Autodesk Fusion 360 part; units mm, degrees
sketch "Sketch1" plane through (0, 0, 0) normal (0, 0, 1) x (1, 0, 0)
  line L0 (68.541, -12.5) -> (-110, -12.5) construction
  line L1 (-20.75, -50) -> (-20.75, 25) construction
  point P0 (-20.75, -12.5)
sketch "Sketch2" plane through (0, 0, 0) normal (0, 0, 1) x (1, 0, 0)
  line L0 (54.25, 7.5) -> (-95.75, 7.5)
  line L1 (-95.75, 7.5) -> (-95.75, -32.5)
  line L2 (-95.75, -32.5) -> (54.25, -32.5)
  line L3 (54.25, -32.5) -> (54.25, 7.5)
  line L4 (54.25, 7.5) -> (-95.75, -32.5) construction
  line L5 (-95.75, 7.5) -> (54.25, -32.5) construction
  line L6 (26.6666, -12.5) -> (38.5, -12.5) construction
  circle A0 centre (32.5833, -12.5) radius 2.75
  line L7 (14, -12.5) -> (2.2, -12.5) construction
  circle A1 centre (8.1, -12.5) radius 2.75
  line L8 (-49.1, -12.5) -> (-52.4, -12.5) construction
  circle A2 centre (-52.4, -12.5) radius 2.75
  line L9 (-73.1, -12.5) -> (-69.8, -12.5) construction
  circle A3 centre (-69.8, -12.5) radius 2.75
  point P0 (-20.75, -12.5)
  dimension "d1" = 150
  dimension "d2" = 40
  dimension "d3" = 5.5
  dimension "d4" = 5.5
  dimension "d5" = 3.3
  dimension "d6" = 5.5
  dimension "d7" = 3.3
  dimension "d8" = 5.5
extrude "Extrude1" add sketch "Sketch2" along normal blind 2.5
sketch "Sketch3" plane through (0, 0, 2.5) normal (0, 0, 1) x (-1, 0, 0)
  circle A0 centre (-32.5833, 12.5) radius 2.75
  circle A1 centre (69.8, 12.5) radius 2.75
  circle A2 centre (-8.1, 12.5) radius 2.75
  circle A3 centre (52.4, 12.5) radius 2.75
  line L0 (-54.25, 32.5) -> (-54.25, -7.5)
  line L1 (-54.25, -7.5) -> (95.75, -7.5)
  line L2 (95.75, -7.5) -> (95.75, 32.5)
  line L3 (95.75, 32.5) -> (-54.25, 32.5)
sketch "Sketch4" plane through (0, 0, 2.5) normal (0, 0, 1) x (-1, 0, 0)
  line L0 (-29.8338, 12.5) -> (-35.3337, 12.5) construction
  line L1 (-39.2087, 4.875) -> (-25.9587, 4.875)
  line L2 (-25.9587, 4.875) -> (-25.9587, 20.125)
  line L3 (-25.9587, 20.125) -> (-39.2087, 20.125)
  line L4 (-39.2087, 20.125) -> (-39.2087, 4.875)
  line L5 (-39.2087, 4.875) -> (-25.9587, 20.125) construction
  line L6 (-25.9587, 4.875) -> (-39.2087, 20.125) construction
  line L7 (-41.2087, 2.875) -> (-23.9587, 2.875)
  line L8 (-23.9587, 2.875) -> (-23.9587, 22.125)
  line L9 (-23.9587, 22.125) -> (-41.2087, 22.125)
  line L10 (-41.2087, 22.125) -> (-41.2087, 2.875)
  line L11 (-41.2087, 2.875) -> (-23.9587, 22.125) construction
  line L12 (-23.9587, 2.875) -> (-41.2087, 22.125) construction
  line L13 (-39.2087, 12.5) -> (-39.2087, 9)
  line L14 (-39.2087, 9) -> (-41.2087, 9)
  line L15 (-41.2087, 9) -> (-41.2087, 16)
  line L16 (-41.2087, 16) -> (-39.2087, 16)
  line L17 (-39.2087, 16) -> (-39.2087, 12.5)
  line L18 (-5.35, 12.5) -> (-10.85, 12.5) construction
  line L19 (-14.725, 4.875) -> (-1.475, 4.875)
  line L20 (-1.475, 4.875) -> (-1.475, 20.125)
  line L21 (-1.475, 20.125) -> (-14.725, 20.125)
  line L22 (-14.725, 20.125) -> (-14.725, 4.875)
  line L23 (-14.725, 4.875) -> (-1.475, 20.125) construction
  line L24 (-1.475, 4.875) -> (-14.725, 20.125) construction
  line L25 (-16.725, 2.875) -> (0.525, 2.875)
  line L26 (0.525, 2.875) -> (0.525, 22.125)
  line L27 (0.525, 22.125) -> (-16.725, 22.125)
  line L28 (-16.725, 22.125) -> (-16.725, 2.875)
  line L29 (-16.725, 2.875) -> (0.525, 22.125) construction
  line L30 (0.525, 2.875) -> (-16.725, 22.125) construction
  line L31 (-1.475, 16) -> (-1.475, 9)
  line L32 (0.525, 16) -> (0.525, 9)
  line L33 (0.525, 9) -> (-1.475, 9)
  line L34 (0.525, 16) -> (-1.475, 16)
  line L35 (55.15, 12.5) -> (49.65, 12.5) construction
  line L36 (45.775, 4.875) -> (59.025, 4.875)
  line L37 (59.025, 4.875) -> (59.025, 20.125)
  line L38 (59.025, 20.125) -> (45.775, 20.125)
  line L39 (45.775, 20.125) -> (45.775, 4.875)
  line L40 (45.775, 4.875) -> (59.025, 20.125) construction
  line L41 (59.025, 4.875) -> (45.775, 20.125) construction
  line L42 (61.025, 22.125) -> (43.775, 22.125)
  line L43 (43.775, 22.125) -> (43.775, 2.875)
  line L44 (43.775, 2.875) -> (61.025, 2.875)
  line L45 (61.025, 22.125) -> (43.775, 2.875) construction
  line L46 (43.775, 22.125) -> (61.025, 2.875) construction
  line L47 (72.55, 12.5) -> (67.05, 12.5) construction
  line L48 (63.175, 4.875) -> (76.425, 4.875)
  line L49 (76.425, 4.875) -> (76.425, 20.125)
  line L50 (76.425, 20.125) -> (63.175, 20.125)
  line L51 (63.175, 20.125) -> (63.175, 4.875)
  line L52 (63.175, 4.875) -> (76.425, 20.125) construction
  line L53 (76.425, 4.875) -> (63.175, 20.125) construction
  line L54 (61.175, 2.875) -> (78.425, 2.875)
  line L55 (78.425, 2.875) -> (78.425, 22.125)
  line L56 (78.425, 22.125) -> (61.175, 22.125)
  line L57 (61.175, 2.875) -> (78.425, 22.125) construction
  line L58 (78.425, 2.875) -> (61.175, 22.125) construction
  line L59 (61.175, 2.875) -> (61.025, 2.875)
  line L60 (61.175, 22.125) -> (61.025, 22.125)
  line L61 (43.775, 16) -> (43.775, 9)
  line L62 (45.775, 16) -> (45.775, 9)
  line L63 (45.775, 9) -> (43.775, 9)
  line L64 (45.775, 16) -> (43.775, 16)
  line L65 (76.425, 16) -> (76.425, 9)
  line L66 (78.425, 16) -> (78.425, 9)
  line L67 (78.425, 9) -> (76.425, 9)
  line L68 (76.425, 16) -> (78.425, 16)
  point P0 (-32.5837, 12.5)
  point P1 (-32.5837, 12.5)
  point P2 (-8.1, 12.5)
  point P3 (-8.1, 12.5)
  point P4 (-1.475, 12.5)
  point P5 (0.525, 12.5)
  point P6 (52.4, 12.5)
  point P7 (52.4, 12.5)
  point P8 (69.8, 12.5)
  point P9 (69.8, 12.5)
  point P10 (43.775, 12.5)
  point P11 (45.775, 12.5)
  point P12 (76.425, 12.5)
  point P13 (78.425, 12.5)
  dimension "d11" = 13.25
  dimension "d12" = 15.25
  dimension "d13" = 17.25
  dimension "d14" = 19.25
  dimension "d15" = 3.5
  dimension "d16" = 7
  dimension "d17" = 13.25
  dimension "d18" = 15.25
  dimension "d19" = 17.25
  dimension "d20" = 19.25
  dimension "d21" = 7
  dimension "d22" = 7
  dimension "d23" = 13.25
  dimension "d24" = 15.25
  dimension "d25" = 17.25
  dimension "d26" = 19.25
  dimension "d27" = 13.25
  dimension "d28" = 15.25
  dimension "d29" = 17.25
  dimension "d30" = 19.25
  dimension "d31" = 7
  dimension "d32" = 7
  dimension "d33" = 7
  dimension "d34" = 7
extrude "Extrude2" add sketch "Sketch4" along normal blind 12 contours L1 L2 L3 L4 L7 L8 L9 L10 L14 L16 | L19 L20 L21 L22 L25 L26 L27 L28 L33 L34 | L36 L37 L38 L39 L42 L43 L44 L48 L49 L50 L51 L54 L55 L56 L59 L60 L63 L64 L67 L68
sketch "Sketch5" plane through (0, 0, 2.5) normal (0, 0, 1) x (-1, 0, 0)
sketch "Sketch7" plane through (54.25, 0, 0) normal (1, 0, 0) x (0, 1, 0)
  line L0 (-32.5, 0) -> (7.5, 0)
  line L1 (7.5, 0) -> (7.5, 2.5)
  line L2 (7.5, 2.5) -> (-32.5, 2.5)
  line L3 (-32.5, 2.5) -> (-32.5, 0)
  line L4 (-25, 2.5) -> (0, 2.5)
  line L5 (-21.5, 2.5) -> (-3.5, 2.5)
  line L6 (-12.5, 7.5) -> (-3.5, 7.5)
  line L7 (-3.5, 7.5) -> (0, 2.5)
  line L8 (-12.5, 7.5) -> (-21.5, 7.5)
  line L9 (-21.5, 7.5) -> (-25, 2.5)
  line L10 (-12.5, 2.5) -> (-12.5, 7.5) construction
  circle A0 centre (-12.5, 5) radius 1.25
  point P0 (-12.5, 2.5)
  point P1 (-12.5, 2.5)
  dimension "d39" = 25
  dimension "d40" = 18
  dimension "d41" = 2.5
extrude "Extrude3" add sketch "Sketch7" against normal blind 2.5 contours L2 L4 L5 L6 L7 L8 L9
sketch "Sketch8" plane through (-95.75, 0, 0) normal (-1, 0, 0) x (0, -1, 0)
  line L0 (-7.5, 0) -> (32.5, 0)
  line L1 (32.5, 0) -> (32.5, 2.5)
  line L2 (32.5, 2.5) -> (-7.5, 2.5)
  line L3 (-7.5, 2.5) -> (-7.5, 0)
  line L4 (0, 2.5) -> (25, 2.5)
  line L5 (3.5, 7.5) -> (21.5, 7.5)
  line L6 (3.5, 7.5) -> (0, 2.5)
  line L7 (21.5, 7.5) -> (25, 2.5)
  circle A0 centre (12.5, 5) radius 1.25
  point P0 (12.5, 2.5)
  dimension "d44" = 25
  dimension "d46" = 18
  dimension "d47" = 2.5
extrude "Extrude4" add sketch "Sketch8" against normal blind 2.5 contours L2 L4 L5 L6 L7
fillet "Fillet1" radius 1 4 edges at (-94.5, -21.5, 7.5) (-94.5, -25, 2.5) (-94.5, -3.5, 7.5) (-94.5, 0, 2.5)
fillet "Fillet2" radius 1 4 edges at (53, -25, 2.5) (53, -21.5, 7.5) (53, -3.5, 7.5) (53, 0, 2.5)
fillet "Fillet3" radius 0.5 5 edges at (41.2087, -19.0625, 2.5) (32.5837, -22.125, 2.5) (41.2087, -5.9375, 2.5) (32.5837, -2.875, 2.5) (23.9587, -12.5, 2.5)
fillet "Fillet4" radius 0.5 15 edges at (16.725, -12.5, 2.5) (8.1, -2.875, 2.5) (8.1, -22.125, 2.5) (-0.525, -5.9375, 2.5) (-0.525, -19.0625, 2.5) (-52.4, -22.125, 2.5) (-61.1, -22.125, 2.5) (-69.8, -22.125, 2.5) (-78.425, -19.0625, 2.5) (-78.425, -5.9375, 2.5) (-43.775, -19.0625, 2.5) (-43.775, -5.9375, 2.5) (-69.8, -2.875, 2.5) (-61.1, -2.875, 2.5) (-52.4, -2.875, 2.5)
fillet "Fillet5" radius 1 8 edges at (-45.775, -16, 8.5) (-45.775, -9, 8.5) (-76.425, -9, 8.5) (-76.425, -16, 8.5) (1.475, -16, 8.5) (1.475, -9, 8.5) (39.2087, -16, 8.5) (39.2087, -9, 8.5)
extrude "Extrude5" add 1 faces at (54.25, -20.0421, 4.8192) along direction (1, 0, 0) blind 3
extrude "Extrude6" cut 1 faces at (51.75, -20.0421, 4.8192) along direction (1, 0, 0) blind 3
extrude "Extrude7" add 1 faces at (-95.75, -20.0421, 4.8192) along direction (-1, 0, 0) blind 3
extrude "Extrude8" cut 1 faces at (-93.25, -20.0421, 4.8192) along direction (-1, 0, 0) blind 3
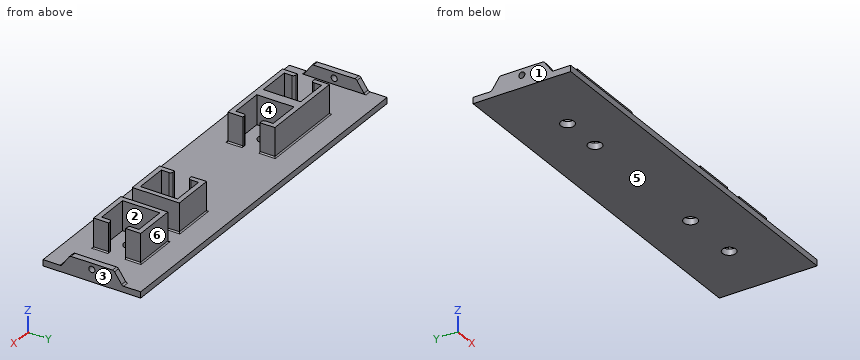
Source: CAD feature listing. Evaluate the final solid. Frame: model axes, mm. Face numbers are marked on the shaded views. A direction names the side the tool comes from. Round coordinates to 2 decimals unless told otherwise and drop trailing zeros. Loops run counter-clockwise (first coordinate to the right, second up) from the corner with the lowest first, then second, coordinate; pieces in that order, holes last. Notation, with made-up numbers: M -6.5,1.5 L 38.5,1.5 A31 ccw 38.5,29.5 Z; hole C 10,65.5 d4. An arc over 180 degrees is marked long. Use a Markdown table: item, result. Add a question column.
1. Ray query, line 1 along Y through (x, z) = (-68, 5.25) (3 decimals); line 2 along Z through (x, y) = (-97.75, -12.5); line 3 along Y through (x, z) = (-52.4, 1.45). Return the intervals inside material, ascending. Write a range as [from, to].
2. Cut plane D-D, the plane x = -34. Output: boundary loops of the cut face in (y, z).
3. Pull-direction query (X, two-part tool) for the marked faces 1, 2 and 3; classes: +X half, -X half, draft (parallel to the pull), parting line (faces both ways), or undercut.
4. Set-up query: the marked faces 4, 5 and 6. Return all of +Z, -Z, +X, -X, +Y, -Y with unobstructed straight access to the full face (end or side cutting, diameter ignored); none if empty.
5. Cut plane C-C, the plane y = -27. Output: boundary loops of the cut face in (x, z), and give its area (3 significant figures).
6. Cut plane A-A, the plane x = 8.1. Output: boundary loops of the cut face in (y, z) (3 decimals), and give its area (3 significant figures).
7. Cut plane B-B, the plane z = 11.25. State how many separate pieces and enclosed holes the cut face has, and give its area (3 significant figures).
8. Contact query for flat-ended pins moving along their axis: pin 1 (3 mm diameter, centred on y = -17.5, z = 9.5, fed in from +X); pin 2 (1.2 mm diameter, centred on x = 41, z = 8, fed in from +Y) (3 decimals); pin 3 (1.5 mm diameter, centred on x = -12, y = -15, fed in from -Z); pin 4 (3 mm diameter, centred on y = -20, z = 10, fed in from -X) (3 decimals). Output: stop coordinate, or through.
Solution:
| question | item | result |
|---|---|---|
| 1 | line 1 | y = [-22.125, -20.125], [-4.875, -2.875] |
| 1 | line 2 | z = [0, 3.75], [6.25, 7.5] |
| 1 | line 3 | y = [-32.5, -15.25], [-9.75, 7.5] |
| 2 | outline | M -32.5,0 L 7.5,0 L 7.5,2.5 L -32.5,2.5 Z |
| 3 | face 1 | -X half |
| 3 | face 2 | undercut |
| 3 | face 3 | +X half |
| 4 | face 4 | +Z |
| 4 | face 5 | -Z, +X, -X, +Y, -Y |
| 4 | face 6 | +Z, +Y |
| 5 | outline | M -98.75,0 L 57.25,0 L 57.25,2.5 L -98.75,2.5 Z |
| 5 | area | 390 mm2 |
| 6 | outline | M -32.5,0 L -15.25,0 L -15.25,2.5 L -20.125,2.5 L -20.125,14.5 L -22.125,14.5 L -22.125,3 A0.5 cw -22.625,2.5 L -32.5,2.5 Z; M -9.75,0 L 7.5,0 L 7.5,2.5 L -2.375,2.5 A0.5 cw -2.875,3 L -2.875,14.5 L -4.875,14.5 L -4.875,2.5 L -9.75,2.5 Z |
| 6 | area | 134 mm2 |
| 7 | separate pieces | 3 |
| 7 | enclosed holes | 0 |
| 7 | area | 465 mm2 |
| 8 | pin 1 | stops at x = 41.21 |
| 8 | pin 2 | stops at y = -2.875 |
| 8 | pin 3 | stops at z = 0 |
| 8 | pin 4 | stops at x = -78.425 |
